```python
from build123d import *

# Parameters (mm, degrees)
BOX_W           = 97
BOX_H           = 66
BOX_DEPTH       = 2
SKETCH015_W     = 97
SKETCH015_H     = 66
SKETCH015_W_2   = 93
SKETCH015_H_2   = 62
PAD012_DEPTH    = 6
SKETCH016_R     = 1.3
PAD013_DEPTH    = 20
SKETCH014_W     = 13
SKETCH014_H     = 27
POCKET004_DEPTH = 4


with BuildPart() as part:
    # Box → Box (join)
    with BuildSketch(Plane.XY):
        with Locations((48.5, 33)):
            Rectangle(BOX_W, BOX_H)
    extrude(amount=BOX_DEPTH)

    # Sketch015 → Pad012 (join)
    with BuildSketch(Plane.XY):
        with Locations((48.5, 33)):
            Rectangle(SKETCH015_W, SKETCH015_H)
        with Locations((48.5, 33)):
            Rectangle(SKETCH015_W_2, SKETCH015_H_2, mode=Mode.SUBTRACT)
    extrude(amount=-PAD012_DEPTH)

    # Sketch016 → Pad013 (join)
    with BuildSketch(Plane.XY):
        with BuildLine():
            Line((27, 57.5), (27, 64))
            Line((27, 64), (32, 64))
            Line((32, 57.5), (32, 64))
            ThreePointArc((27, 57.5), (29.5, 55), (32, 57.5))
        make_face()
        with Locations((29.5, 57.5)):
            Circle(SKETCH016_R, mode=Mode.SUBTRACT)
        with BuildLine():
            Line((85, 57.5), (85, 64))
            Line((90, 64), (85, 64))
            Line((90, 57.5), (90, 64))
            ThreePointArc((85, 57.5), (87.5, 55), (90, 57.5))
        make_face()
        with Locations((87.5, 57.5)):
            Circle(SKETCH016_R, mode=Mode.SUBTRACT)
        with BuildLine():
            ThreePointArc((90, 8.5), (87.5, 11), (85, 8.5))
            Line((85, 8.5), (85, 2))
            Line((85, 2), (90, 2))
            Line((90, 8.5), (90, 2))
        make_face()
        with Locations((87.5, 8.5)):
            Circle(SKETCH016_R, mode=Mode.SUBTRACT)
        with BuildLine():
            Line((27, 8.5), (27, 2))
            Line((32, 2), (27, 2))
            Line((32, 8.5), (32, 2))
            ThreePointArc((32, 8.5), (29.5, 11), (27, 8.5))
        make_face()
        with Locations((29.5, 8.5)):
            Circle(SKETCH016_R, mode=Mode.SUBTRACT)
    extrude(amount=-PAD013_DEPTH)

    # Sketch014 → Pocket004 (cut)
    with BuildSketch(Plane.XY.offset(2)):
        Polygon((48.5, 62), (48.5, 35), (43.5, 35), (43.5, 62), (46, 62), align=None)
        with Locations((27, 48.5)):
            Rectangle(SKETCH014_W, SKETCH014_H)
        with Locations((65, 48.5)):
            Rectangle(SKETCH014_W, SKETCH014_H)
    extrude(amount=-POCKET004_DEPTH, mode=Mode.SUBTRACT)


solid = part.part
```
Can you work these out from the model? Positions are in its coordinate system, mm. A direction names the side the tool comes from. Coordinates: 2 decimals unless noted, no trailing zeros. Write each loop counter-clockwise with the first axis right and the second up, starting at its lowest first coordinate (ties: lowest second). Pieces come first, ordered by that corner, then holes. Notation, with made-up numbers: M 78,72.25 L 104,72.25 A6 ccw 104,83.25 Z; hole C -25,48 d1. An arc over 180 degrees is marked long. Answer as CSV lines item,"result".
Item 1: Imagine slicing it at B-B on y = 39. List the corners of the cut face in (x, z) for me, plus the area to 3 significant figures.
Geometry results:
outline,"M 0,-6 L 2,-6 L 2,0 L 20.5,0 L 20.5,2 L 0,2 Z; M 33.5,0 L 43.5,0 L 43.5,2 L 33.5,2 Z; M 48.5,0 L 58.5,0 L 58.5,2 L 48.5,2 Z; M 71.5,0 L 95,0 L 95,-6 L 97,-6 L 97,2 L 71.5,2 Z"
area,"156 mm2"
Item 2: Imagine slicing it at C-C on x = 29.5. List the corners of the cut face in (y, z) for me.
Geometry results:
outline,"M 0,-6 L 2,-6 L 2,-20 L 7.2,-20 L 7.2,0 L 9.8,0 L 9.8,-20 L 11,-20 L 11,0 L 35,0 L 35,2 L 0,2 Z; M 55,-20 L 56.2,-20 L 56.2,-2 L 55,-2 Z; M 58.8,-20 L 64,-20 L 64,-6 L 66,-6 L 66,2 L 62,2 L 62,-2 L 58.8,-2 Z"
Item 3: Please list where these lines run through material, in increasing order: line 1 along Y through (x, z) = (87.5, -5.25); line 2 along Y through (x, z) = (87.5, -11.75); line 3 along Y through (x, z) = (19.5, -2.25).
Geometry results:
line 1,"y = 0 to 7.2, 9.8 to 11, 55 to 56.2, 58.8 to 66"
line 2,"y = 2 to 7.2, 9.8 to 11, 55 to 56.2, 58.8 to 64"
line 3,"y = 0 to 2, 64 to 66"
Item 4: Imagine slicing it at A-A on z = -17. List the corners of the cut face in (x, y) for me.
Geometry results:
outline,"M 27,2 L 32,2 L 32,8.5 A2.5 ccw 27,8.5 Z; M 27,57.5 A2.5 ccw 32,57.5 L 32,64 L 27,64 Z; M 85,2 L 90,2 L 90,8.5 A2.5 ccw 85,8.5 Z; M 85,57.5 A2.5 ccw 90,57.5 L 90,64 L 85,64 Z; hole C 29.5,8.5 d2.6; hole C 29.5,57.5 d2.6; hole C 87.5,8.5 d2.6; hole C 87.5,57.5 d2.6"
Item 5: Imagine slicing it at D-D on x = 52. List the corners of the cut face in (y, z) for me.
Geometry results:
outline,"M 0,-6 L 2,-6 L 2,0 L 64,0 L 64,-6 L 66,-6 L 66,2 L 0,2 Z"
Item 6: On a 3-axis mill with a long thin cutter (end or side, diameter ignored), from which of +Z, -Z, +X, -X, +Y, -Y can I reach the whole of each face in a straight line? I mean faces 4 (the flat face through (20.5, 48, 1)), 5 (the flat face through (87, 58, 0)), 6 (the flat face through (48, 0, -2)), 7 (the flat face through (29, 64, -13)), 8 (the flat face through (30, 2, -13)). Say none if no direction works.
Geometry results:
face 4,"+Z, -Z"
face 5,"-Z"
face 6,"+Z, -Z, +X, -X, -Y"
face 7,"-Z, +X, -X, +Y"
face 8,"-Z, +X, -X, -Y"
Item 7: I'm going to push flat-ended pins straight in: P1, Ø7, axis at y = 4, z = -7, coming from the +X side; P2, Ø5.5, axis at x = 86.5, z = -12.5, coming from the -Y side; P3, Ø3.5, axis at x = 29.5, y = 57.5, coming from the +Z side; P4, Ø1.5, axis at x = 10.5, y = 49.5, coming from the -Z side. Where does each tip first touch, or does it pass through?
Geometry results:
P1,"stops at x = 97"
P2,"stops at y = 2"
P3,"stops at z = -2"
P4,"stops at z = 0"
Item 8: We'd pull the mould along X, two halves only. Please class faces 1 (the flat face through (26.9, 62, 0.5)), 2 (the flat face through (34, 1, -6)), 3 (the flat face through (48.5, 49, 1)): +X half, -X half, draft (parallel to the pull), parting line (faces both ways), or undercut.
Geometry results:
face 1,"undercut"
face 2,"draft"
face 3,"undercut"
